from build123d import *

# Parameters (mm, degrees)
SKETCH1_R           = 3.175
BOSS_EXTRUDE1_DEPTH = 6.35
FILLET1_R           = 3.175


with BuildPart() as part:
    # Sketch1 → Boss-Extrude1 (new body)
    with BuildSketch(Plane(origin=(0, 0, 0), x_dir=(1, 0, 0), z_dir=(0, 1, 0))):
        with BuildLine():
            ThreePointArc((55.88, 63.5), (0, 7.62), (-55.88, 63.5))
            Line((-55.88, 63.5), (-65.405, 63.5))
            Line((-65.405, 63.5), (-101.231750934, -37.066318412))
            ThreePointArc((-101.231750934, -37.066318412), (-101.50726052, -38.116025925), (-101.6, -39.197317183))
            Line((-101.6, -39.197317183), (-101.6, -63.5))
            Line((-101.6, -63.5), (101.6, -63.5))
            Line((101.6, -63.5), (101.6, -39.197317183))
            ThreePointArc((101.6, -39.197317183), (101.50726052, -38.116025925), (101.231750934, -37.066318412))
            Line((101.231750934, -37.066318412), (65.405, 63.5))
            Line((65.405, 63.5), (55.88, 63.5))
        make_face()
        with Locations(Location((-63.5, -50.8, 0), (0, 0, 270))):
            Circle(SKETCH1_R, mode=Mode.SUBTRACT)
        with Locations(Location((-25.4, -50.8, 0), (0, 0, 270))):
            Circle(SKETCH1_R, mode=Mode.SUBTRACT)
        with BuildLine():
            Line((-30.492459165, -38.1), (-82.485514384, -38.1))
            ThreePointArc((-82.485514384, -38.1), (-87.67465411, -35.409962965), (-88.467265319, -29.61900123))
            Line((-88.467265319, -29.61900123), (-67.620951247, 28.896968093))
            ThreePointArc((-67.620951247, 28.896968093), (-62.60882158, 33.04150393), (-56.579551543, 30.602954379))
            Line((-56.579551543, 30.602954379), (-24.890648803, -28.759645393))
            ThreePointArc((-24.890648803, -28.759645393), (-25.046761241, -35.016018084), (-30.492459165, -38.1))
        make_face(mode=Mode.SUBTRACT)
        with BuildLine():
            ThreePointArc((-5.299041163, -38.1), (-8.565059247, -37.195697924), (-10.900851525, -34.740354607))
            Line((-10.900851525, -34.740354607), (-24.84623891, -8.616557995))
            ThreePointArc((-24.84623891, -8.616557995), (-24.197984845, -1.653196967), (-17.541381774, 0.491159744))
            ThreePointArc((-17.541381774, 0.491159744), (-0.588821605, -1.902349454), (16.404084946, 0.185546499))
            ThreePointArc((16.404084946, 0.185546499), (22.928583423, -1.961591642), (23.68255589, -8.788802499))
            Line((23.68255589, -8.788802499), (10.859081809, -34.577314678))
            ThreePointArc((10.859081809, -34.577314678), (8.517567892, -37.14796018), (5.173240471, -38.1))
            Line((5.173240471, -38.1), (-5.299041163, -38.1))
        make_face(mode=Mode.SUBTRACT)
        with Locations(Location((25.4, -50.8, 0), (0, 0, 270))):
            Circle(SKETCH1_R, mode=Mode.SUBTRACT)
        with Locations(Location((63.5, -50.8, 0), (0, 0, 270))):
            Circle(SKETCH1_R, mode=Mode.SUBTRACT)
        with BuildLine():
            Line((67.620951247, 28.896968093), (88.467265319, -29.61900123))
            ThreePointArc((88.467265319, -29.61900123), (87.67465411, -35.409962965), (82.485514384, -38.1))
            Line((82.485514384, -38.1), (29.423726477, -38.1))
            ThreePointArc((29.423726477, -38.1), (23.956198754, -34.979340583), (23.862621229, -28.684611212))
            Line((23.862621229, -28.684611212), (56.428690976, 30.395444829))
            ThreePointArc((56.428690976, 30.395444829), (62.481851802, 33.059810636), (67.620951247, 28.896968093))
        make_face(mode=Mode.SUBTRACT)
    extrude(amount=BOSS_EXTRUDE1_DEPTH)

    # Fillet1
    fillet1_edges = [part.edges().sort_by_distance(p)[0] for p in [
        (-65.405, 3.175, -63.5),
        (65.405, 3.175, -63.5),
    ]]
    fillet(fillet1_edges, radius=FILLET1_R)


solid = part.part
Model file for the job. Use its own axes, mm. A direction names the side the tool comes from. Give positions to 0.01 mm unless a question says otherwise; leave off trailing zeros. Loops run counter-clockwise (first coordinate to the right, second up) from the corner with the lowest first, then second, coordinate; pieces in that order, holes last.
1) Saw through at D-D (z = -10.5). Write the cut outline in (x, y), plus the area to 3 significant figures.
2) Saw through at A-A (z = 50.8). Write the cut outline in (x, y) (3 decimals), plus the area to 3 significant figures.
3) Saw through at C-C (x = -75). Write the cut outline in (y, z).
4) Wall check: line 1 (X direction, y = 4.25, z = 50.8) (3 decimals); line 2 (Z direction, x = 0, y = 2.25) (3 decimals); line 3 (X direction, y = 1.75, z = 8). Give the ranges that are in metal, low to high.
5) Pull direction X, two halves, no side cores. Call faces 1 (the flat face through (83.94, 3.13, -11.47)), 2 (the flat face through (-83.45, 3.13, -12.85)), 3 (the flat face through (-17.776, 3.131, 21.861)): +X half, -X half, draft (parallel to the pull), parting line (faces both ways), or undercut.
6) Flat gauge pins, fed straight in: pin 1 Ø2 at (y, z) = (4.5, 11) entering from -X; pin 2 Ø3 at (y, z) = (4, 29) entering from -X; pin 3 Ø5.5 at (x, z) = (-63.5, 50.8) entering from +Y; pin 4 Ø1 at (y, z) = (1.5, 12) entering from -X. Where does each tip first touch, or does it go through?
7) Saw through at B-B (z = -47). Write the cut outline in (x, y).
8) Tool access for faces 4 (the flat face through (-101.6, 3, 51)), 5 (the cylindrical face through (-87.625, 3.131, 35.479)): list every direction of +Z, -Z, +X, -X, +Y, -Y with a clear straight run to the whole face (end or side of a thin tool).
Answer block:
1. outline: (-84.29, 0) - (-74.17, 0) - (-74.17, 6.35) - (-84.29, 6.35) - close; (-45.85, 0) - (-17.71, 0) - (-17.71, 6.35) - (-45.85, 6.35) - close; (17.71, 0) - (45.46, 0) - (45.46, 6.35) - (17.71, 6.35) - close; (74.17, 0) - (84.29, 0) - (84.29, 6.35) - (74.17, 6.35) - close
1. area: 483 mm2
2. outline: (-101.6, 0) - (-66.675, 0) - (-66.675, 6.35) - (-101.6, 6.35) - close; (-60.325, 0) - (-28.575, 0) - (-28.575, 6.35) - (-60.325, 6.35) - close; (-22.225, 0) - (22.225, 0) - (22.225, 6.35) - (-22.225, 6.35) - close; (28.575, 0) - (60.325, 0) - (60.325, 6.35) - (28.575, 6.35) - close; (66.675, 0) - (101.6, 0) - (101.6, 6.35) - (66.675, 6.35) - close
2. area: 1,130 mm2
3. outline: (0, -36.57) - (6.35, -36.57) - (6.35, -8.18) - (0, -8.18) - close; (0, 38.1) - (6.35, 38.1) - (6.35, 63.5) - (0, 63.5) - close
4. line 1: x = -101.6 to -66.675, -60.325 to -28.575, -22.225 to 22.225, 28.575 to 60.325, 66.675 to 101.6
4. line 2: z = -7.62 to 1.905, 38.1 to 63.5
4. line 3: x = -90.88 to -80.77, -35.97 to -25.13, 24.01 to 35.26, 80.77 to 90.88
5. face 1: +X half
5. face 2: -X half
5. face 3: undercut
6. pin 1: stops at x = -92.3
6. pin 2: stops at x = -98.89
6. pin 3: passes through
6. pin 4: stops at x = -92.48
7. outline: (-71.28, 0) - (-53.39, 0) - (-53.39, 6.35) - (-71.28, 6.35) - close; (53.39, 0) - (71.28, 0) - (71.28, 6.35) - (53.39, 6.35) - close
8. face 4: +Z, -Z, -X, +Y, -Y
8. face 5: +Y, -Y
